The model under review builds one solid part; all positions refer to its coordinate system, in mm. Face numbers are marked on the shaded views. A direction names the side the tool comes from. Round coordinates to 2 decimals unless told otherwise and drop trailing zeros. Order: outer loops, then holes, each group sorted by start corner. A loop starts at its lowest first (then second) coordinate and runs counter-clockwise, first axis right, second up.
```python
from build123d import *

# Parameters (mm, degrees)
SKETCH1_W           = 35
SKETCH1_H           = 55
BOSS_EXTRUDE1_DEPTH = 3
SKETCH2_W           = 5
SKETCH2_H           = 5
BOSS_EXTRUDE2_DEPTH = 7
CUT_EXTRUDE1_REACH  = 45.362
FILLET1_R           = 2.5
SKETCH4_W           = 5
SKETCH4_H           = 5
BOSS_EXTRUDE3_DEPTH = 16.61764706
CUT_EXTRUDE2_REACH  = 51.887
FILLET2_R           = 2.5


with BuildPart() as part:
    # Sketch1 → Boss-Extrude1 (new body)
    with BuildSketch(Plane.XY):
        Rectangle(SKETCH1_W, SKETCH1_H)
    extrude(amount=BOSS_EXTRUDE1_DEPTH)

    # Sketch2 → Boss-Extrude2 (add)
    with BuildSketch(Plane.XY.offset(3)):
        with Locations((-12, 25)):
            Rectangle(SKETCH2_W, SKETCH2_H)
        with Locations((12, 25)):
            Rectangle(SKETCH2_W, SKETCH2_H)
        with Locations((-12, -25)):
            Rectangle(SKETCH2_W, SKETCH2_H)
        with Locations((12, -25)):
            Rectangle(SKETCH2_W, SKETCH2_H)
    extrude(amount=BOSS_EXTRUDE2_DEPTH)

    # Cut-Extrude1: up to this face of the body (flat: up to its plane)
    cut_extrude1_end = Plane(part.part.faces().sort_by_distance((14.5, 25, 6.5))[0])
    # Sketch3 → Cut-Extrude1 (cut, up to the picked face)
    with BuildSketch(Plane.ZY.offset(14.5), mode=Mode.PRIVATE) as cut_extrude1_sk1:
        with BuildLine():
            ThreePointArc((8, 25), (6.957766147, 26.428443263), (5.279399793, 25.871857291))
            Line((5.279399793, 25.871857291), (7.720600207, 24.128142709))
            ThreePointArc((7.720600207, 24.128142709), (7.928443263, 24.542233853), (8, 25))
        make_face()
    cut_extrude1_tool1 = split(extrude(cut_extrude1_sk1.sketch, amount=-CUT_EXTRUDE1_REACH, mode=Mode.PRIVATE), bisect_by=cut_extrude1_end, keep=Keep.BOTH, mode=Mode.PRIVATE)
    # Sketch3 → Cut-Extrude1 (cut, up to the picked face)
    with BuildSketch(Plane.ZY.offset(14.5), mode=Mode.PRIVATE) as cut_extrude1_sk2:
        with BuildLine():
            Line((7.720600207, 24.128142709), (5.279399793, 25.871857291))
            ThreePointArc((5.279399793, 25.871857291), (5.628142709, 23.779399793), (7.720600207, 24.128142709))
        make_face()
    cut_extrude1_tool2 = split(extrude(cut_extrude1_sk2.sketch, amount=-CUT_EXTRUDE1_REACH, mode=Mode.PRIVATE), bisect_by=cut_extrude1_end, keep=Keep.BOTH, mode=Mode.PRIVATE)
    # Sketch3 → Cut-Extrude1 (cut, up to the picked face)
    with BuildSketch(Plane.ZY.offset(14.5), mode=Mode.PRIVATE) as cut_extrude1_sk3:
        with BuildLine():
            ThreePointArc((8, 25), (6.957766147, 26.428443263), (5.279399793, 25.871857291))
            Line((5.279399793, 25.871857291), (7.720600207, 24.128142709))
            ThreePointArc((7.720600207, 24.128142709), (7.928443263, 24.542233853), (8, 25))
        make_face()
    cut_extrude1_tool3 = split(extrude(cut_extrude1_sk3.sketch, amount=-CUT_EXTRUDE1_REACH, mode=Mode.PRIVATE), bisect_by=cut_extrude1_end, keep=Keep.BOTH, mode=Mode.PRIVATE)
    # Sketch3 → Cut-Extrude1 (cut, up to the picked face)
    with BuildSketch(Plane.ZY.offset(14.5), mode=Mode.PRIVATE) as cut_extrude1_sk4:
        with BuildLine():
            Line((7.720600207, 24.128142709), (5.279399793, 25.871857291))
            ThreePointArc((5.279399793, 25.871857291), (5.628142709, 23.779399793), (7.720600207, 24.128142709))
        make_face()
    cut_extrude1_tool4 = split(extrude(cut_extrude1_sk4.sketch, amount=-CUT_EXTRUDE1_REACH, mode=Mode.PRIVATE), bisect_by=cut_extrude1_end, keep=Keep.BOTH, mode=Mode.PRIVATE)
    # Sketch3 → Cut-Extrude1 (cut, up to the picked face)
    with BuildSketch(Plane.ZY.offset(14.5), mode=Mode.PRIVATE) as cut_extrude1_sk5:
        with BuildLine():
            ThreePointArc((8, -25), (6.957766147, -23.571556737), (5.279399793, -24.128142709))
            Line((5.279399793, -24.128142709), (7.720600207, -25.871857291))
            ThreePointArc((7.720600207, -25.871857291), (7.928443263, -25.457766147), (8, -25))
        make_face()
    cut_extrude1_tool5 = split(extrude(cut_extrude1_sk5.sketch, amount=-CUT_EXTRUDE1_REACH, mode=Mode.PRIVATE), bisect_by=cut_extrude1_end, keep=Keep.BOTH, mode=Mode.PRIVATE)
    # Sketch3 → Cut-Extrude1 (cut, up to the picked face)
    with BuildSketch(Plane.ZY.offset(14.5), mode=Mode.PRIVATE) as cut_extrude1_sk6:
        with BuildLine():
            Line((7.720600207, -25.871857291), (5.279399793, -24.128142709))
            ThreePointArc((5.279399793, -24.128142709), (5.628142709, -26.220600207), (7.720600207, -25.871857291))
        make_face()
    cut_extrude1_tool6 = split(extrude(cut_extrude1_sk6.sketch, amount=-CUT_EXTRUDE1_REACH, mode=Mode.PRIVATE), bisect_by=cut_extrude1_end, keep=Keep.BOTH, mode=Mode.PRIVATE)
    # Sketch3 → Cut-Extrude1 (cut, up to the picked face)
    with BuildSketch(Plane.ZY.offset(14.5), mode=Mode.PRIVATE) as cut_extrude1_sk7:
        with BuildLine():
            ThreePointArc((8, -25), (6.957766147, -23.571556737), (5.279399793, -24.128142709))
            Line((5.279399793, -24.128142709), (7.720600207, -25.871857291))
            ThreePointArc((7.720600207, -25.871857291), (7.928443263, -25.457766147), (8, -25))
        make_face()
    cut_extrude1_tool7 = split(extrude(cut_extrude1_sk7.sketch, amount=-CUT_EXTRUDE1_REACH, mode=Mode.PRIVATE), bisect_by=cut_extrude1_end, keep=Keep.BOTH, mode=Mode.PRIVATE)
    # Sketch3 → Cut-Extrude1 (cut, up to the picked face)
    with BuildSketch(Plane.ZY.offset(14.5), mode=Mode.PRIVATE) as cut_extrude1_sk8:
        with BuildLine():
            Line((7.720600207, -25.871857291), (5.279399793, -24.128142709))
            ThreePointArc((5.279399793, -24.128142709), (5.628142709, -26.220600207), (7.720600207, -25.871857291))
        make_face()
    cut_extrude1_tool8 = split(extrude(cut_extrude1_sk8.sketch, amount=-CUT_EXTRUDE1_REACH, mode=Mode.PRIVATE), bisect_by=cut_extrude1_end, keep=Keep.BOTH, mode=Mode.PRIVATE)
    add(cut_extrude1_tool1.solids().sort_by(Axis((-14.5, 25.518039, 6.870028), (1, 0, 0)))[0], mode=Mode.SUBTRACT)
    add(cut_extrude1_tool2.solids().sort_by(Axis((-14.5, 24.481961, 6.129972), (1, 0, 0)))[0], mode=Mode.SUBTRACT)
    add(cut_extrude1_tool3.solids().sort_by(Axis((-14.5, 25.518039, 6.870028), (1, 0, 0)))[0], mode=Mode.SUBTRACT)
    add(cut_extrude1_tool4.solids().sort_by(Axis((-14.5, 24.481961, 6.129972), (1, 0, 0)))[0], mode=Mode.SUBTRACT)
    add(cut_extrude1_tool5.solids().sort_by(Axis((-14.5, -24.481961, 6.870028), (1, 0, 0)))[0], mode=Mode.SUBTRACT)
    add(cut_extrude1_tool6.solids().sort_by(Axis((-14.5, -25.518039, 6.129972), (1, 0, 0)))[0], mode=Mode.SUBTRACT)
    add(cut_extrude1_tool7.solids().sort_by(Axis((-14.5, -24.481961, 6.870028), (1, 0, 0)))[0], mode=Mode.SUBTRACT)
    add(cut_extrude1_tool8.solids().sort_by(Axis((-14.5, -25.518039, 6.129972), (1, 0, 0)))[0], mode=Mode.SUBTRACT)

    # Fillet1
    fillet1_edges = [part.edges().sort_by_distance(p)[0] for p in [
        (12, -27.5, 10),
        (12, -22.5, 10),
        (-12, -27.5, 10),
        (-12, -22.5, 10),
    ]]
    fillet(fillet1_edges, radius=FILLET1_R - 0.0001)  # a hair under: the kernel refuses the full size

    # Sketch4 → Boss-Extrude3 (add)
    with BuildSketch(Plane.XY.offset(10)):
        with Locations((-12, 25)):
            Rectangle(SKETCH4_W, SKETCH4_H)
        with Locations((12, 25)):
            Rectangle(SKETCH4_W, SKETCH4_H)
    extrude(amount=BOSS_EXTRUDE3_DEPTH)

    # Cut-Extrude2: up to this face of the body (flat: up to its plane)
    cut_extrude2_end = Plane(part.part.faces().sort_by_distance((14.5, 25, 15.337843498))[0])
    # Sketch5 → Cut-Extrude2 (cut, up to the picked face)
    with BuildSketch(Plane.ZY.offset(14.5), mode=Mode.PRIVATE) as cut_extrude2_sk1:
        with BuildLine():
            ThreePointArc((24.61764706, 25), (23.575413207, 26.428443263), (21.897046853, 25.871857291))
            Line((21.897046853, 25.871857291), (24.338247267, 24.128142709))
            ThreePointArc((24.338247267, 24.128142709), (24.546090323, 24.542233853), (24.61764706, 25))
        make_face()
    cut_extrude2_tool1 = split(extrude(cut_extrude2_sk1.sketch, amount=-CUT_EXTRUDE2_REACH, mode=Mode.PRIVATE), bisect_by=cut_extrude2_end, keep=Keep.BOTH, mode=Mode.PRIVATE)
    # Sketch5 → Cut-Extrude2 (cut, up to the picked face)
    with BuildSketch(Plane.ZY.offset(14.5), mode=Mode.PRIVATE) as cut_extrude2_sk2:
        with BuildLine():
            Line((24.338247267, 24.128142709), (21.897046853, 25.871857291))
            ThreePointArc((21.897046853, 25.871857291), (22.245789769, 23.779399793), (24.338247267, 24.128142709))
        make_face()
    cut_extrude2_tool2 = split(extrude(cut_extrude2_sk2.sketch, amount=-CUT_EXTRUDE2_REACH, mode=Mode.PRIVATE), bisect_by=cut_extrude2_end, keep=Keep.BOTH, mode=Mode.PRIVATE)
    # Sketch5 → Cut-Extrude2 (cut, up to the picked face)
    with BuildSketch(Plane.ZY.offset(14.5), mode=Mode.PRIVATE) as cut_extrude2_sk3:
        with BuildLine():
            ThreePointArc((24.61764706, 25), (23.575413207, 26.428443263), (21.897046853, 25.871857291))
            Line((21.897046853, 25.871857291), (24.338247267, 24.128142709))
            ThreePointArc((24.338247267, 24.128142709), (24.546090323, 24.542233853), (24.61764706, 25))
        make_face()
    cut_extrude2_tool3 = split(extrude(cut_extrude2_sk3.sketch, amount=-CUT_EXTRUDE2_REACH, mode=Mode.PRIVATE), bisect_by=cut_extrude2_end, keep=Keep.BOTH, mode=Mode.PRIVATE)
    # Sketch5 → Cut-Extrude2 (cut, up to the picked face)
    with BuildSketch(Plane.ZY.offset(14.5), mode=Mode.PRIVATE) as cut_extrude2_sk4:
        with BuildLine():
            Line((24.338247267, 24.128142709), (21.897046853, 25.871857291))
            ThreePointArc((21.897046853, 25.871857291), (22.245789769, 23.779399793), (24.338247267, 24.128142709))
        make_face()
    cut_extrude2_tool4 = split(extrude(cut_extrude2_sk4.sketch, amount=-CUT_EXTRUDE2_REACH, mode=Mode.PRIVATE), bisect_by=cut_extrude2_end, keep=Keep.BOTH, mode=Mode.PRIVATE)
    add(cut_extrude2_tool1.solids().sort_by(Axis((-14.5, 25.518039, 23.487675), (1, 0, 0)))[0], mode=Mode.SUBTRACT)
    add(cut_extrude2_tool2.solids().sort_by(Axis((-14.5, 24.481961, 22.747619), (1, 0, 0)))[0], mode=Mode.SUBTRACT)
    add(cut_extrude2_tool3.solids().sort_by(Axis((-14.5, 25.518039, 23.487675), (1, 0, 0)))[0], mode=Mode.SUBTRACT)
    add(cut_extrude2_tool4.solids().sort_by(Axis((-14.5, 24.481961, 22.747619), (1, 0, 0)))[0], mode=Mode.SUBTRACT)

    # Fillet2
    fillet2_edges = [part.edges().sort_by_distance(p)[0] for p in [
        (12, 22.5, 26.61764706),
        (12, 27.5, 26.61764706),
        (-12, 22.5, 26.61764706),
        (-12, 27.5, 26.61764706),
    ]]
    fillet(fillet2_edges, radius=FILLET2_R - 0.0001)  # a hair under: the kernel refuses the full size


solid = part.part
```
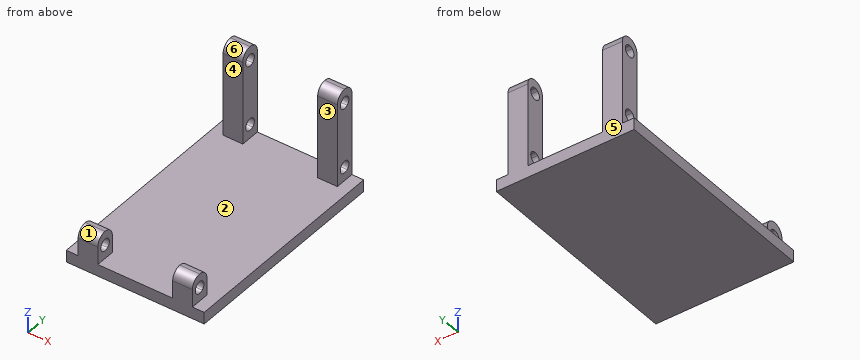
(1) Consider section C-C (x = 0). Write out the cut boundary in (y, z).
Data:
outline: (-27.5, 0) - (27.5, 0) - (27.5, 3) - (-27.5, 3) - close
(2) For the marked faces 1 and 2, list the 3-axis set-ups (+Z, -Z, +X, -X, +Y, -Y) from which the entire face can be reached by the end or side of a thin tool; tool diameter is ignored.
Data:
face 1: +Z, +X, -X, -Y
face 2: +Z
(3) Insertion check: pin 1 (2.5 mm diameter, centred on x = -12, z = 17, fed in from -Y); pin 2 (4 mm diameter, centred on y = 25, z = 9.5, fed in from +X); pin 3 (5.5 mm diameter, centred on y = -24.5, z = 7.5, fed in from -X). Each pin has a flat end and moves straight along its axis. Give the tip position at first contact, or say it passes through.
Data:
pin 1: stops at y = 22.5
pin 2: stops at x = 14.5
pin 3: stops at x = -14.5
(4) Consider section A-A (z = 6.5). State how many separate pieces and enclosed holes the cut face has, and give its area (3 significant figures).
Data:
separate pieces: 8
enclosed holes: 0
area: 40.0 mm2
(5) Draft analysis for pull direction Y (two halves, no side actions). For the marked faces 3, 4, 5 and 6, state which applies: pulls with the +Y half, pulls with the -Y half, needs draft (parallel to the pull), parting line crosses it, or undercut.
Data:
face 3: undercut
face 4: undercut
face 5: pulls with the +Y half
face 6: pulls with the -Y half
(6) To check wall thickness, follow probe 1 along Y at (x, z) = (13, 14.5); probe 2 along Z at (x, y) = (2, 21); probe 3 along Y at (x, z) = (-11, 4). State the ranges of each line that lie inside material, in increasing order.
Data:
probe 1: y = 22.5 to 27.5
probe 2: z = 0 to 3
probe 3: y = -27.5 to -22.5, 22.5 to 27.5
(7) Consider section B-B (y = -11). Write out the cut boundary in (x, z).
Data:
outline: (-17.5, 0) - (17.5, 0) - (17.5, 3) - (-17.5, 3) - close
